Here's the drawing with two shaded views (mm, measured from the low corner). I have some questions. Coordinates: 2 decimals unless noted, no trailing zeros. Loops run counter-clockwise (first coordinate to the right, second up) from the corner with the lowest first, then second, coordinate; pieces in that order, holes last. Notation, with made-up numbers: (63, -23.75) - (85, -23.75) arc R15 cw to (85, 5.25) - close; hole circle Ø1 at (-39.5, -20). An arc over 180 degrees is marked (long way). One line per item, written item: value. Start each with the question number.
(1) If we section it at C-C on x = 55.5: Write out the boundary of the cut face in (y, z).
(2) If we section it at A-A on y = 0.8: Write out the boundary of the cut face in (x, z), then the cut area to 3 significant figures.
(3) I'm going to push a flat-ended pin straight in: P1, Ø5, axis at x = 71.5, z = 4, coming from the -Y side. Where does the tip first touch, or does it pass through?
(4) If we section it at B-B on z = 25: Write out the boundary of the cut face in (x, y).
(5) If I drill on line 1 along X through (y, z) = (1.3, 10.5) (1 decimal); line 2 along X through (y, z) = (2.45, 32); line 3 along Z through (x, y) = (51, 2.55), over which ranges is the centre line in solid material (lowest first)? Write a range as from..to.
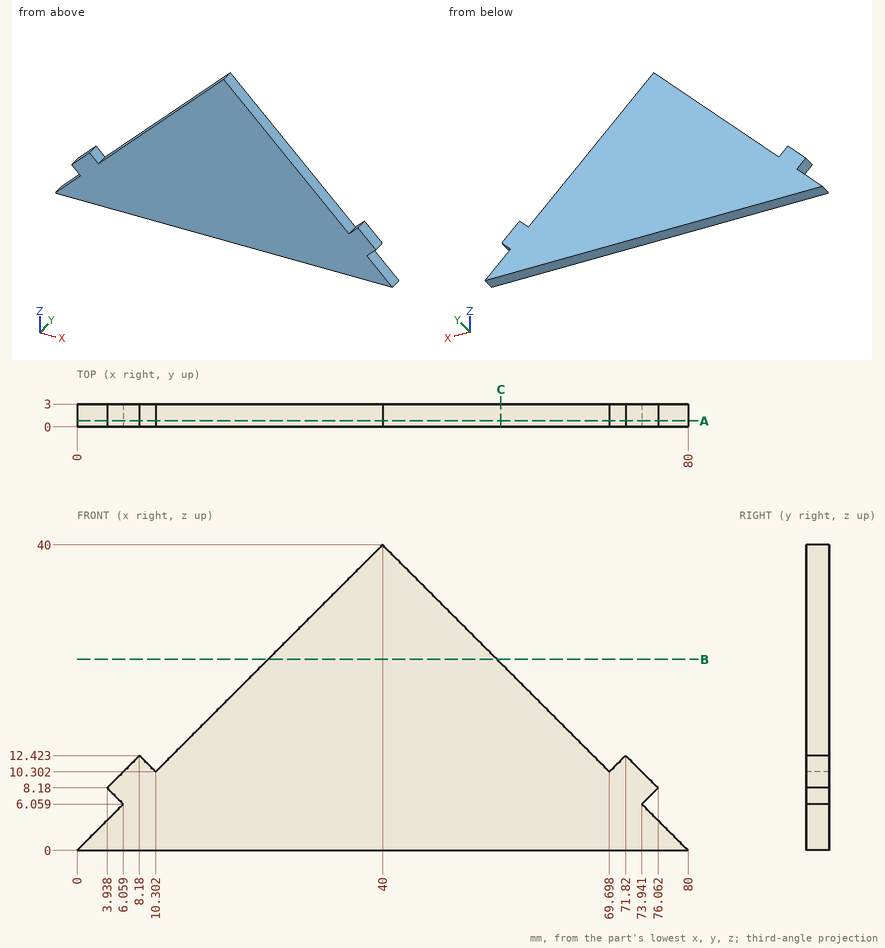
Values:
1. outline: (0, 0) - (3, 0) - (3, 24.5) - (0, 24.5) - close
2. outline: (0, 0) - (80, 0) - (73.94, 6.06) - (76.06, 8.18) - (71.82, 12.42) - (69.7, 10.3) - (40, 40) - (10.3, 10.3) - (8.18, 12.42) - (3.94, 8.18) - (6.06, 6.06) - close
2. area: 1,640 mm2
3. P1: stops at y = 0
4. outline: (25, 0) - (55, 0) - (55, 3) - (25, 3) - close
5. line 1: x = 6.3..10.1, 10.5..69.5, 69.9..73.7
5. line 2: x = 32..48
5. line 3: z = 0..29
